Verification items for the finished model (mm, model axes). Give positions to 0.01 mm unless a question says otherwise; leave off trailing zeros. Answer as a JSON object with one key per item and string values. Group by question number.
(1) Mould release check, pull along X, two halves, no side actions. Record for faces 1 (the face through (150, 10, 37)), 2 (the face through (0, 20, 37)), 3 (the face through (100, 10, 37)): +X half, -X half, draft (parallel to the pull), parting line (faces both ways), or undercut.
(2) Thickness scan on line 1 (Z direction, x = 2, y = 20); line 2 (Z direction, x = 156.75, y = 20); line 3 (Y direction, x = 18.5, z = 70). Record the ranges inside material, lowest first.
(3) Section check A-A (y = 30). Count the separate pieces of the cut face and the enclosed holes in it, then the cut area to 3 significant figures.
(4) Depth check by flat-ended pin: pin 1 Ø4 at (x, z) = (40, 28) entering from +Y; pin 2 Ø2 at (x, y) = (18.5, 5) entering from +Z. Enter the tip coordinate at first touch or a pass-through.
```python
from build123d import *

# Parameters (mm, degrees)
BOSS_EXTRUDE1_DEPTH = 74.5
SKETCH2_R           = 1.25
CUT_EXTRUDE1_DEPTH  = 10
SKETCH3_R           = 1.25
CUT_EXTRUDE2_DEPTH  = 10
SKETCH4_R           = 1.25
CUT_EXTRUDE3_DEPTH  = 15
CUT_EXTRUDE4_START  = -15
SKETCH5_R           = 1.25
CUT_EXTRUDE4_DEPTH  = 15


with BuildPart() as part:
    # Sketch1 → Boss-Extrude1 (new body)
    with BuildSketch(Plane.XY):
        Polygon((0, 0), (0, 40), (6, 40), (7.5, 10), (12.5, 10), (14, 40), (16, 40), (17.5, 10), (22.5, 10), (24, 40), (26, 40), (27.5, 10), (32.5, 10), (34, 40), (36, 40), (37.5, 10), (42.5, 10), (44, 40), (46, 40), (47.5, 10), (52.5, 10), (54, 40), (56, 40), (57.5, 10), (62.5, 10), (64, 40), (66, 40), (67.5, 10), (72.5, 10), (74, 40), (76, 40), (77.5, 10), (82.5, 10), (84, 40), (86, 40), (87.5, 10), (92.5, 10), (94, 40), (96, 40), (97.5, 10), (102.5, 10), (104, 40), (106, 40), (107.5, 10), (112.5, 10), (114, 40), (116, 40), (117.5, 10), (122.5, 10), (124, 40), (126, 40), (127.5, 10), (132.5, 10), (134, 40), (136, 40), (137.5, 10), (142.5, 10), (144, 40), (146, 40), (147.5, 10), (152.5, 10), (154, 40), (160, 40), (160, 0), align=None)
    extrude(amount=BOSS_EXTRUDE1_DEPTH)

    # Sketch2 → Cut-Extrude1 (cut)
    with BuildSketch(Plane(origin=(160, 0, 0), x_dir=(0, 0, -1), z_dir=(1, 0, 0))):
        with Locations((-64.5, 20)):
            Circle(SKETCH2_R)
        with Locations((-10, 20)):
            Circle(SKETCH2_R)
    extrude(amount=-CUT_EXTRUDE1_DEPTH, mode=Mode.SUBTRACT)

    # Sketch3 → Cut-Extrude2 (cut)
    with BuildSketch(Plane.ZY):
        with Locations((20, 20)):
            Circle(SKETCH3_R)
        with Locations((54.5, 20)):
            Circle(SKETCH3_R)
    extrude(amount=-CUT_EXTRUDE2_DEPTH, mode=Mode.SUBTRACT)

    # Sketch4 → Cut-Extrude3 (cut)
    with BuildSketch(Plane.XY.offset(74.5)):
        with Locations((18.5, 5)):
            Circle(SKETCH4_R)
        with Locations((120, 5)):
            Circle(SKETCH4_R)
    extrude(amount=-CUT_EXTRUDE3_DEPTH, mode=Mode.SUBTRACT)

    # Sketch5 → Cut-Extrude4 (cut)
    with BuildSketch(Plane(origin=(0, 0, 0), x_dir=(-1, 0, 0), z_dir=(0, 0, -1)).offset(CUT_EXTRUDE4_START)):
        with Locations(Location((-120, 5, 0), (0, 0, 180))):
            Circle(SKETCH5_R)
        with Locations(Location((-18.5, 5, 0), (0, 0, 180))):
            Circle(SKETCH5_R)
    extrude(amount=CUT_EXTRUDE4_DEPTH, mode=Mode.SUBTRACT)


solid = part.part
```
Solutions:
{
 "1": {"face 1": "undercut", "face 2": "-X half", "face 3": "undercut"},
 "2": {"line 1": "z = 0 to 18.75, 21.25 to 53.25, 55.75 to 74.5", "line 2": "z = 0 to 8.75, 11.25 to 63.25, 65.75 to 74.5", "line 3": "y = 0 to 3.75, 6.25 to 10"},
 "3": {"separate pieces": "16", "enclosed holes": "0", "area": "4,100 mm2"},
 "4": {"pin 1": "stops at y = 10", "pin 2": "stops at z = 59.5"}
}
